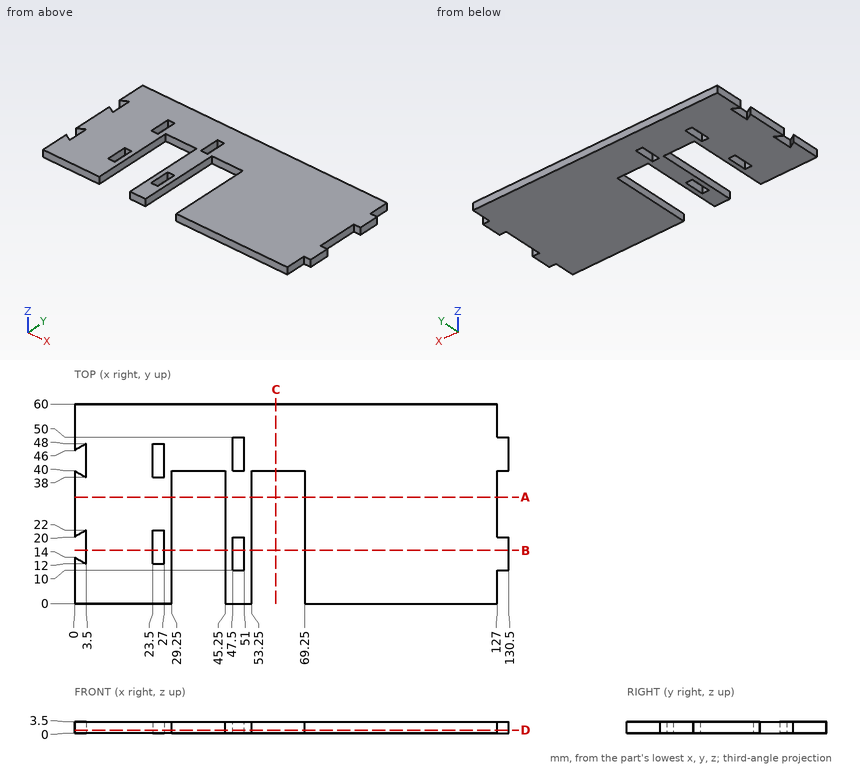
Study the drawing (mm; zero at the part's minimum x, y, z) and answer. Give positions to 0.01 mm unless a question says otherwise; leave off trailing zeros. Loops run counter-clockwise (first coordinate to the right, second up) from the corner with the lowest first, then second, coordinate; pieces in that order, holes last. Notation, with made-up numbers: (11.25, 54.25) - (39.25, 54.25) arc R27 cw to (39.25, 82.25) - close; hole circle Ø11 at (31.25, 65.5). An arc over 180 degrees is marked (long way). Return JSON: item names as keys, results as strings. Group by question number.
1. Given pin 1 Ø1.8 at (y, z) = (18, 1) entering from -X; pin 2 Ø1.8 at (y, z) = (30.5, 1.5) entering from +X, each flat-ended and moving along its own axis, determine where each tip first touches the part or whether it passes through.
2. Straight lines are drawn through the part: line 1 (X direction, y = 17, z = 0.5); line 2 (Y direction, x = 25.5, z = 3.1); line 3 (X direction, y = 24, z = 1.05). For each, find the intervals that lie inside material, in ascending order. Write a range as [from, to].
3. Find section D-D (z = 1). State how many separate pieces and enclosed holes the cut face has, then the cut area to 3 significant figures.
4. Find section A-A (y = 32). Write down the section's boundary in (x, z), then the cut area to 4 significant figures.
5. Find section C-C (x = 60.5). Write down the section's boundary in (y, z).
6. Find section B-B (y = 16). Write down the section's boundary in (x, z), then the cut area to 3 significant figures.
Verdict:
{
 "1": {"pin 1": "stops at x = 3.5", "pin 2": "stops at x = 127"},
 "2": {"line 1": "x = [3.5, 23.5], [27, 29.25], [45.25, 47.5], [51, 53.25], [69.25, 130.5]", "line 2": "y = [0, 12], [22, 38], [48, 60]", "line 3": "x = [0, 29.25], [45.25, 53.25], [69.25, 127]"},
 "3": {"separate pieces": "1", "enclosed holes": "4", "area": "6,210 mm^2"},
 "4": {"outline": "(0, 0) - (29.25, 0) - (29.25, 3.5) - (0, 3.5) - close; (45.25, 0) - (53.25, 0) - (53.25, 3.5) - (45.25, 3.5) - close; (69.25, 0) - (127, 0) - (127, 3.5) - (69.25, 3.5) - close", "area": "332.5 mm^2"},
 "5": {"outline": "(40, 0) - (60, 0) - (60, 3.5) - (40, 3.5) - close"},
 "6": {"outline": "(3.5, 0) - (23.5, 0) - (23.5, 3.5) - (3.5, 3.5) - close; (27, 0) - (29.25, 0) - (29.25, 3.5) - (27, 3.5) - close; (45.25, 0) - (47.5, 0) - (47.5, 3.5) - (45.25, 3.5) - close; (51, 0) - (53.25, 0) - (53.25, 3.5) - (51, 3.5) - close; (69.25, 0) - (130.5, 0) - (130.5, 3.5) - (69.25, 3.5) - close", "area": "308 mm^2"}
}
